from build123d import *

# Parameters (mm, degrees)
SKETCH1_R           = 4.2
BOSS_EXTRUDE1_DEPTH = 16.51
SKETCH2_R           = 1.2
BOSS_EXTRUDE2_DEPTH = 0.8
SKETCH3_R           = 0.45
BOSS_EXTRUDE3_DEPTH = 3.92
FILLET3_R           = 0.05
FILLET4_R           = 0.1


with BuildPart() as part:
    # Sketch1 → Boss-Extrude1 (new body)
    with BuildSketch(Plane(origin=(0, 0, 0), x_dir=(1, 0, 0), z_dir=(0, 1, 0))):
        Circle(SKETCH1_R)
    extrude(amount=BOSS_EXTRUDE1_DEPTH)

    # Sketch2 → Boss-Extrude2 (add)
    with BuildSketch(Plane(origin=(0, 16.51, 0), x_dir=(1, 0, 0), z_dir=(0, 1, 0))):
        Circle(SKETCH2_R)
    extrude(amount=BOSS_EXTRUDE2_DEPTH)

    # Sketch3 → Boss-Extrude3 (add)
    with BuildSketch(Plane(origin=(0, 17.31, 0), x_dir=(1, 0, 0), z_dir=(0, 1, 0))):
        Circle(SKETCH3_R)
    extrude(amount=BOSS_EXTRUDE3_DEPTH)

    # Fillet3
    fillet3_edges = [part.edges().sort_by_distance(p)[0] for p in [
        (-0.45, 17.31, 0),
        (-1.2, 16.51, 0),
        (-1.2, 17.31, 0),
    ]]
    fillet(fillet3_edges, radius=FILLET3_R)

    # Fillet4
    fillet4_edges = [part.edges().sort_by_distance(p)[0] for p in [
        (-4.2, 16.51, 0),
    ]]
    fillet(fillet4_edges, radius=FILLET4_R)


solid = part.part
Model file for the job. Use its own axes, mm. A direction names the side the tool comes from. Give positions to 0.01 mm unless a question says otherwise; leave off trailing zeros. Loops run counter-clockwise (first coordinate to the right, second up) from the corner with the lowest first, then second, coordinate; pieces in that order, holes last.
1) Saw through at C-C (y = 19.25). Write the cut outline in (x, z), plus the area to 3 significant figures.
2) Wall check: line 1 (Y direction, x = 1.5, z = 2.75); line 2 (Y direction, x = -0.75, z = 0.75); line 3 (X direction, y = 17.25, z = 0). Give the ranges that are in metal, low to high.
3) Saw through at B-B (z = 0). Write the cut outline in (x, y).
4) Saw through at A-A (x = 0). Write the cut outline in (y, z), plus the area to 3 significant figures.
5) Tool access for faces 1 (the flat face through (0, 21.23, 0)), 2 (the flat face through (-1, 16.51, 1)): list every direction of +Z, -Z, +X, -X, +Y, -Y with a clear straight run to the whole face (end or side of a thin tool).
6) Saw through at D-D (y = 17). Write the cut outline in (x, z), plus the area to 3 significant figures.
7) Flat gauge pins, fed straight in: pin 1 Ø3 at (x, z) = (2.5, -2.5) entering from +Y; pin 2 Ø2 at (x, y) = (1.5, 13.5) entering from -Z; pin 3 Ø4 at (x, y) = (2.5, 15) entering from +Z. Where does each tip first touch, or does it go through?
Answer block:
1. outline: circle Ø0.9 at (0, 0)
1. area: 0.636 mm2
2. line 1: y = 0 to 16.51
2. line 2: y = 0 to 17.31
2. line 3: x = -1.2 to 1.2
3. outline: (-4.2, 0) - (4.2, 0) - (4.2, 16.41) arc R0.1 ccw to (4.1, 16.51) - (1.25, 16.51) arc R0.05 cw to (1.2, 16.56) - (1.2, 17.26) arc R0.05 ccw to (1.15, 17.31) - (0.5, 17.31) arc R0.05 cw to (0.45, 17.36) - (0.45, 21.23) - (-0.45, 21.23) - (-0.45, 17.36) arc R0.05 cw to (-0.5, 17.31) - (-1.15, 17.31) arc R0.05 ccw to (-1.2, 17.26) - (-1.2, 16.56) arc R0.05 cw to (-1.25, 16.51) - (-4.1, 16.51) arc R0.1 ccw to (-4.2, 16.41) - close
4. outline: (0, -4.2) - (16.41, -4.2) arc R0.1 ccw to (16.51, -4.1) - (16.51, -1.25) arc R0.05 cw to (16.56, -1.2) - (17.26, -1.2) arc R0.05 ccw to (17.31, -1.15) - (17.31, -0.5) arc R0.05 cw to (17.36, -0.45) - (21.23, -0.45) - (21.23, 0.45) - (17.36, 0.45) arc R0.05 cw to (17.31, 0.5) - (17.31, 1.15) arc R0.05 ccw to (17.26, 1.2) - (16.56, 1.2) arc R0.05 cw to (16.51, 1.25) - (16.51, 4.1) arc R0.1 ccw to (16.41, 4.2) - (0, 4.2) - close
4. area: 144 mm2
5. face 1: +Z, -Z, +X, -X, +Y
5. face 2: +Y
6. outline: circle Ø2.4 at (0, 0)
6. area: 4.52 mm2
7. pin 1: stops at y = 16.51
7. pin 2: stops at z = -4.17
7. pin 3: stops at z = 4.17
